from build123d import *

# Parameters (mm, degrees)
F0_W      = 120.65
F0_H      = 76.2
F2_DEPTH  = 38.1
F1_W      = 69.85
F1_H      = 101.6
F3_DEPTH  = 38.1
F4_R      = 3.7467551061
F5_DEPTH  = 38.1
F6_W      = 25.4
F6_H      = 19.05
F7_DEPTH  = 203.2
F8_W      = 6.35
F8_H      = 50.8
F8_H_2    = 76.2
F9_DEPTH  = 47.626
F11_DEPTH = 38.1
F12_R     = 5.08


with BuildPart() as f2:
    # F0 (on Top) → F2 (new body, symmetric)
    with BuildSketch(Plane.XY):
        Rectangle(F0_W, F0_H)
    extrude(amount=F2_DEPTH, both=True)

    # F1 (on face) → F3 (cut, symmetric)
    with BuildSketch(Plane.XY):
        with Locations((0, -50.8)):
            Rectangle(F1_W, F1_H)
    extrude(amount=F3_DEPTH, both=True, mode=Mode.SUBTRACT)

    # F4 (on face) → F5 (cut, symmetric)
    with BuildSketch(Plane.YZ.offset(60.325)):
        with Locations((-16.3753926754, 0)):
            Circle(F4_R)
    extrude(amount=F5_DEPTH, both=True, mode=Mode.SUBTRACT)

    # F6 (on face) → F7 (join)
    with BuildSketch(Plane(origin=(0, 38.1, 0), x_dir=(-1, 0, 0), z_dir=(0, 1, 0))):
        with Locations((47.625, 0)):
            Rectangle(F6_W, F6_H)
    extrude(amount=F7_DEPTH)

    # F8 (on face) → F9 (cut, through all)
    with BuildSketch(Plane.XY.offset(9.525)):
        with Locations((-47.625, 196.85)):
            Rectangle(F8_W, F8_H)
        with Locations((-47.625, 114.3)):
            Rectangle(F8_W, F8_H_2)
    extrude(amount=-F9_DEPTH, mode=Mode.SUBTRACT)

    # F10 (on Top) → F11 (join, symmetric)
    with BuildSketch(Plane.XY):
        Polygon((-29.2977448553, -18.0150475353), (-34.9880978465, -10.1638017222), (-35.0601263344, -27.8110988438), align=None)
    extrude(amount=F11_DEPTH, both=True)

    # F12
    f12_edges = [f2.edges().sort_by_distance(p)[0] for p in [
        (60.325, -38.1, 0),
        (60.325, 0, 38.1),
        (60.325, 38.1, 0),
        (60.325, 0, -38.1),
        (0, 38.1, 38.1),
        (-60.325, 38.1, 23.8125),
        (-60.325, 38.1, -23.8125),
        (0, 38.1, -38.1),
        (-60.325, 0, 38.1),
        (-60.325, -38.1, 0),
        (-60.325, 0, -38.1),
        (34.925, -38.1, 0),
        (-34.925, -27.581384, 0),
        (-32.111372, -22.798216, 38.1),
        (-29.297745, -18.015048, 0),
        (-32.111372, -22.798216, -38.1),
        (0, 0, 38.1),
        (0, 0, -38.1),
        (47.625, -38.1, 38.1),
        (47.625, -38.1, -38.1),
        (-47.625, -38.1, 38.1),
        (-47.625, -38.1, -38.1),
        (-34.925, -5.12543, 38.1),
        (-32.111372, -14.132954, 38.1),
        (-34.925, -32.840692, 38.1),
        (34.925, -19.05, 38.1),
        (-34.925, -32.840692, -38.1),
    ]]
    fillet(f12_edges, radius=F12_R)


solid = f2.part
Here's how the part is built. I have some questions about the finished solid (model axes, mm). A direction names the side the tool comes from. Round coordinates to 2 decimals unless told otherwise and drop trailing zeros. Loops run counter-clockwise (first coordinate to the right, second up) from the corner with the lowest first, then second, coordinate; pieces in that order, holes last.
1. For P1, Ø12, axis at x = 20.5, z = -16, coming from the +Y side; P2, Ø21, axis at y = 205, z = 1, coming from the +X side (3 decimals); P3, Ø12.5, axis at x = -53, y = 129, coming from the -Z side (3 decimals), each with a flat end and sliding along its axis, tell me the tip position at first contact or that it passes through.
Answer list:
P1: stops at y = 38.1
P2: stops at x = -34.925
P3: stops at z = -9.525
2. If we section it at B-B on y = 148: Write out the boundary of the cut face in (x, z) (3 decimals), plus the area to 3 significant figures.
Answer list:
outline: (-60.325, -9.525) - (-50.8, -9.525) - (-50.8, 9.525) - (-60.325, 9.525) - close; (-44.45, -9.525) - (-34.925, -9.525) - (-34.925, 9.525) - (-44.45, 9.525) - close
area: 363 mm2
3. We'd pull the mould along Y, two halves only. Please class faces 4 (the face through (-33.829, -22.862, 36.572)), 5 (the face through (-1, 8, 38.1)), 6 (the face through (-48, 76.2, 0)): +Y half, -Y half, draft (parallel to the pull), parting line (faces both ways), or undercut.
Answer list:
face 4: -Y half
face 5: draft
face 6: undercut
4. If we section it at C-C on z = -16: Write out the boundary of the cut face in (x, y) (3 decimals).
Answer list:
outline: (-60.325, -33.02) arc R5.08 ccw to (-55.245, -38.1) - (-34.925, -38.1) - (-34.925, -28.965) arc R5.08 cw to (-34.224, -26.389) - (-30.983, -20.88) arc R5.08 ccw to (-31.249, -15.323) - (-34.925, -10.251) - (-34.925, 0) - (34.925, 0) - (34.925, -33.02) arc R5.08 ccw to (40.005, -38.1) - (55.245, -38.1) arc R5.08 ccw to (60.325, -33.02) - (60.325, 33.02) arc R5.08 ccw to (55.245, 38.1) - (-55.245, 38.1) arc R5.08 ccw to (-60.325, 33.02) - close
5. Which directions (+Z, -Z, +X, -X, +Y, -Y) give clear straight access to the entire face, cutting with the end or side of a thin tool? Please do faces 1 (the face through (36.45, -13.7, 36.65)), 2 (the face through (-34.925, -34, 0)), 3 (the face through (-58.88, 36.57, 21.11)).
Answer list:
face 1: +Z, -Y
face 2: +Z, -Z, -Y
face 3: +Z, -X, +Y
6. If we section it at D-D on x = -27: Write out the boundary of the cut face in (y, z).
Answer list:
outline: (0, -33.02) arc R5.08 ccw to (5.08, -38.1) - (33.02, -38.1) arc R5.08 ccw to (38.1, -33.02) - (38.1, 33.02) arc R5.08 ccw to (33.02, 38.1) - (5.08, 38.1) arc R5.08 ccw to (0, 33.02) - close
7. If we section it at A-A on z = 0: Count the separate pieces of the cut face and the enclosed holes in it, plus the area to 3 significant figures.
Answer list:
separate pieces: 2
enclosed holes: 2
area: 10,700 mm2
8. If I drill on line 1 along X through (y, z) = (-8, -5.5) (3 decimals); line 2 along X through (y, z) = (179, -2.5) (3 decimals); line 3 along X through (y, z) = (168, 5.5) (3 decimals), over which ranges is the centre line in solid material (lowest first)?
Answer list:
line 1: x = -60.325 to -34.925, 34.925 to 60.325
line 2: x = -60.325 to -50.8, -44.45 to -34.925
line 3: x = -60.325 to -34.925
